Check sheet for the drawn part. Datum: minimum x, y, z corner. Units: mm. A direction names the side the tool comes from. Give positions to 0.01 mm unless a question says otherwise; leave off trailing zeros. Loops run counter-clockwise (first coordinate to the right, second up) from the corner with the lowest first, then second, coordinate; pieces in that order, holes last. Notation, with made-up numbers: (3.25, 5) - (36.25, 5) arc R20 ccw to (36.25, 44) - close; hole circle Ø9 at (29, 27). An arc over 180 degrees is marked (long way). Use one line per item in the form item = value.
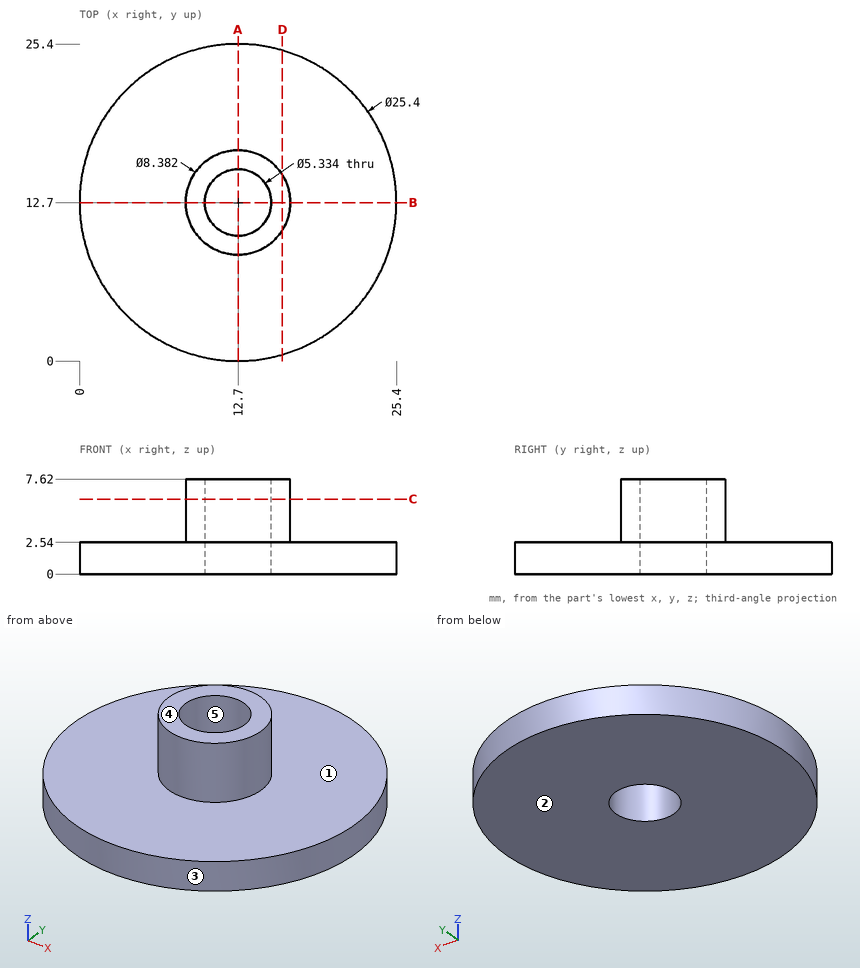
1. Tool access check on the marked faces 1 and 2. Record the directions out of +Z, -Z, +X, -X, +Y, -Y that give a thin tool (end or side, any length) a straight path to the whole face; none if there is none.
Result set:
face_1 = +Z
face_2 = -Z, +X, -X, +Y, -Y
2. Depth check by flat-ended pin: pin 1 Ø4 at (x, z) = (21, 3) entering from -Y; pin 2 Ø4 at (x, y) = (4, 12.5) entering from +Z. Enter the tip coordinate at first touch or a pass-through.
Result set:
pin_1 = 1.7
pin_2 = 2.54
3. Draft check along Y on the marked faces 3, 4 and 5. Enter one of: released by +Y, released by -Y, zero draft, split by the parting line, or undercut.
Result set:
face_3 = split by the parting line
face_4 = zero draft
face_5 = undercut
4. Scan lines: probe 1 along X at (y, z) = (12.7, 4.75); probe 2 along Z at (x, y) = (20.5, 16.75). Record each from-to range of solid material in increasing order.
Result set:
probe_1 = 8.51 to 10.03, 15.37 to 16.89
probe_2 = 0 to 2.54
5. Section check A-A, the plane x = 12.7. Record the cut outline in (y, z), then the cut area to 3 significant figures.
Result set:
outline = (0, 0) - (10.03, 0) - (10.03, 7.62) - (8.51, 7.62) - (8.51, 2.54) - (0, 2.54) - close; (15.37, 0) - (25.4, 0) - (25.4, 2.54) - (16.89, 2.54) - (16.89, 7.62) - (15.37, 7.62) - close
area = 66.5 mm²
6. Section check D-D, the plane x = 16.25. Record the cut outline in (y, z), then the cut area to 3 significant figures.
Result set:
outline = (0.51, 0) - (24.89, 0) - (24.89, 2.54) - (14.93, 2.54) - (14.93, 7.62) - (10.47, 7.62) - (10.47, 2.54) - (0.51, 2.54) - close
area = 84.6 mm²
7. Section check C-C, the plane z = 6. Record the cut outline in (x, y), then the cut area to 3 significant figures.
Result set:
outline = circle Ø8.38 at (12.7, 12.7); hole circle Ø5.33 at (12.7, 12.7)
area = 32.8 mm²
